Print and shaded views of the part. All mm, measured from the part's lowest x, y and z. Round coordinates to 2 decimals unless told otherwise and drop trailing zeros. Loops run counter-clockwise (first coordinate to the right, second up) from the corner with the lowest first, then second, coordinate; pieces in that order, holes last. Notation, with made-up numbers: (48.25, -2) - (80.25, -2) arc R24 ccw to (80.25, 33) - close; hole circle Ø4 at (42.5, 52.25). An arc over 180 degrees is marked (long way). Use one line per item in the form item = value.
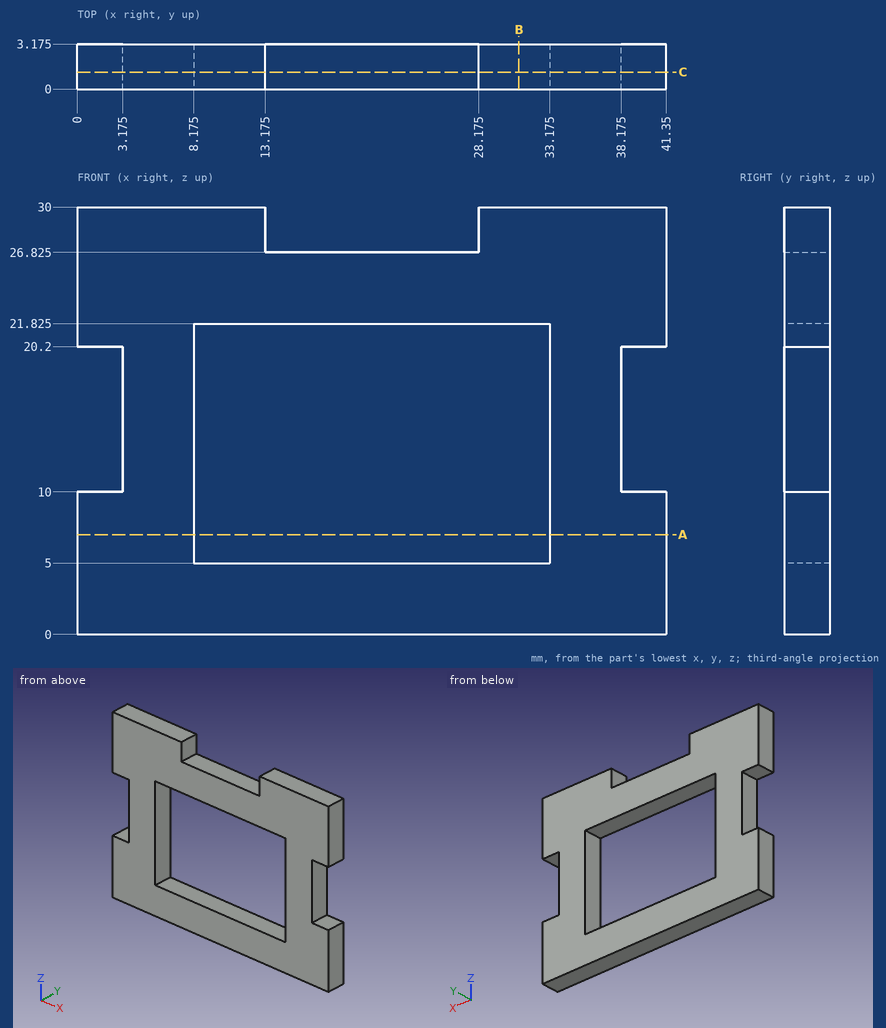
1) Slice it at B-B (x = 31). Write the cut outline in (y, z) (3 decimals).
Report:
outline = (0, 0) - (3.175, 0) - (3.175, 5) - (0, 5) - close; (0, 21.825) - (3.175, 21.825) - (3.175, 30) - (0, 30) - close
2) Flat gauge pins, fed straight in: pin 1 (1.6 mm diameter, centred on x = 18.5, y = 1, fed in from +Z) (3 decimals); pin 2 (1.5 mm diameter, centred on y = 2.5, z = 11.5, fed in from -X) (3 decimals); pin 3 (1 mm diameter, centred on y = 1, z = 28, fed in from -X); pin 4 (1 mm diameter, centred on y = 1, z = 16.5, fed in from +X) (3 decimals). Where does each tip first touch, or does it go through?
Report:
pin_1 = 26.825
pin_2 = 3.175
pin_3 = 0
pin_4 = 38.175
3) Drill centre lines: probe 1 along Z at (x, y) = (24.5, 1.65) (3 decimals); probe 2 along X at (y, z) = (2.65, 19) (3 decimals); probe 3 along X at (y, z) = (0.7, 28.25) (3 decimals). Where is each one in solid material? Low to high.
Report:
probe_1 = 0 to 5, 21.825 to 26.825
probe_2 = 3.175 to 8.175, 33.175 to 38.175
probe_3 = 0 to 13.175, 28.175 to 41.35
4) Slice it at C-C (y = 1.2). Write the cut outline in (x, z) (3 decimals), plus the area to 3 significant figures.
Report:
outline = (0, 0) - (41.35, 0) - (41.35, 10) - (38.175, 10) - (38.175, 20.2) - (41.35, 20.2) - (41.35, 30) - (28.175, 30) - (28.175, 26.825) - (13.175, 26.825) - (13.175, 30) - (0, 30) - (0, 20.2) - (3.175, 20.2) - (3.175, 10) - (0, 10) - close; hole (8.175, 5) - (33.175, 5) - (33.175, 21.825) - (8.175, 21.825) - close
area = 707 mm^2
5) Slice it at A-A (z = 7). Write the cut outline in (x, y) (3 decimals), plus the area to 3 significant figures.
Report:
outline = (0, 0) - (8.175, 0) - (8.175, 3.175) - (0, 3.175) - close; (33.175, 0) - (41.35, 0) - (41.35, 3.175) - (33.175, 3.175) - close
area = 51.9 mm^2
